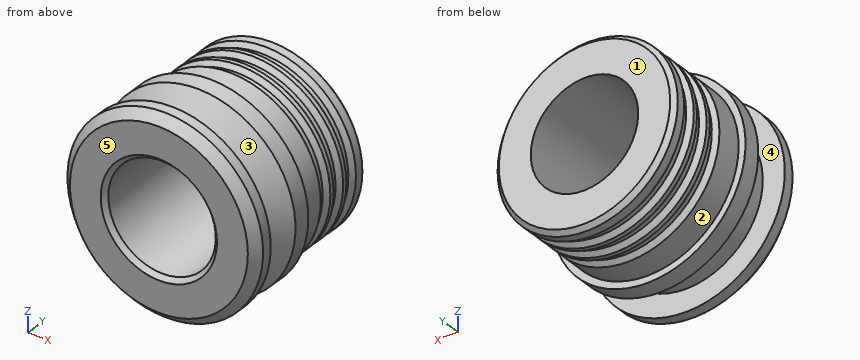
```python
from build123d import *

# Parameters (mm, degrees)
CHAMFER_1_SIZE = 1
CHAMFER_2_SIZE = 0.5
CHAMFER_3_SIZE = 0.5


with BuildPart() as part:
    # 스케치1 → 회전1 (revolve)
    with BuildSketch(Plane(origin=(0, 0, 0), x_dir=(0, 0, -1), z_dir=(1, 0, 0))):
        Polygon((6.1, 0), (6.1, 18.2), (10.225, 18.2), (10.225, 16.7), (9.725, 16.200000049), (9.725, 15.700000049), (10.225, 15.2), (10.225, 14.7), (9.725, 14.200000049), (9.725, 13.700000049), (10.225, 13.2), (10.225, 12.7), (9.725, 12.200000049), (9.725, 11.700000049), (10.225, 11.2), (10.225, 8.2), (11, 8.2), (11, 6.2), (8.6, 4.2), (8.6, 2.2), (11.1, 2.2), (11.1, 0), align=None)
    revolve(axis=Axis((0, 0, 0), (0, 1, 0)))

    # 모따기1
    chamfer_1_edges = [part.edges().sort_by_distance(p)[0] for p in [
        (0, 0, 11.1),
    ]]
    chamfer(chamfer_1_edges, length=CHAMFER_1_SIZE)

    # 모따기2
    chamfer_2_edges = [part.edges().sort_by_distance(p)[0] for p in [
        (0, 18.2, 10.225),
    ]]
    chamfer(chamfer_2_edges, length=CHAMFER_2_SIZE)

    # 모따기3
    chamfer_3_edges = [part.edges().sort_by_distance(p)[0] for p in [
        (0, 0, 6.1),
    ]]
    chamfer(chamfer_3_edges, length=CHAMFER_3_SIZE)


solid = part.part
```
CAD build for the part. Positions are in the model's coordinates, mm. Face numbers are marked on the shaded views. A direction names the side the tool comes from. Round coordinates to 2 decimals unless told otherwise and drop trailing zeros. Write each loop counter-clockwise with the first axis right and the second up, starting at its lowest first coordinate (ties: lowest second). Pieces come first, ordered by that corner, then holes.
Item 1: Band-saw the part on A-A on y = 4.75. Write the cut outline in (x, z), then the cut area to 3 significant figures.
Filled in:
outline: circle Ø18.52 at (0, 0); hole circle Ø12.2 at (0, 0)
area: 152 mm2
Item 2: Drop flat-ended pins along their axis: pin 1 Ø1.5 at (x, z) = (-4.5, -0.5) entering from +Y; pin 2 Ø5 at (x, y) = (0, 15) entering from +Z (3 decimals); pin 3 Ø3 at (x, y) = (1.5, 4.5) entering from +Z; pin 4 Ø3 at (y, z) = (5.5, -7) entering from -X. Give the stop position or say it passes through.
Filled in:
pin 1: passes through
pin 2: stops at z = 10.225
pin 3: stops at z = 10.67
pin 4: stops at x = -9.42
Item 3: Mould opens along Y. For the marked faces 1, 2 and 3 say: released by +Y, released by -Y, zero draft, split by the parting line, or undercut.
Filled in:
face 1: released by +Y
face 2: zero draft
face 3: undercut
Item 4: Tool access for the marked faces 4 and 5: list every direction of +Z, -Z, +X, -X, +Y, -Y with a clear straight run to the whole face (end or side of a thin tool).
Filled in:
face 4: none
face 5: +Z, -Z, +X, -X, -Y
Item 5: Drill centre lines: L1, parallel to X at y = 12.75, z = 0 (3 decimals); L2, parallel to Z at x = 0, y = 4.5; L3, parallel to Z at x = -4, y = 5. Where is each one in solid material? Low to high.
Filled in:
L1: x = -10.225 to -6.1, 6.1 to 10.225
L2: z = -8.96 to -6.1, 6.1 to 8.96
L3: z = -8.68 to -4.61, 4.61 to 8.68
Item 6: Band-saw the part on B-B on y = 7.75. Write the cut outline in (x, z), then the cut area to 3 significant figures.
Filled in:
outline: circle Ø22 at (0, 0); hole circle Ø12.2 at (0, 0)
area: 263 mm2
